Build history of the part. All positions in model axes, mm. A direction names the side the tool comes from. Round coordinates to 2 decimals unless told otherwise and drop trailing zeros. Write each loop counter-clockwise with the first axis right and the second up, starting at its lowest first coordinate (ties: lowest second). Pieces come first, ordered by that corner, then holes. Notation, with made-up numbers: (6.25, 36) -> (20.25, 36) arc R23 ccw to (20.25, 63) -> close; hole circle Ø11 at (67.5, -1.75). An arc over 180 degrees is marked (long way). Answer in a Markdown table with one row per item.
```python
from build123d import *
from build123d import SkipClean  # not in build123d's __all__

# Parameters (mm, degrees)
F1_DEPTH = 15.6
F2_R     = 4.15
F3_DEPTH = 2.1


with BuildPart() as f1:
    # F0 (on Top) → F1 (new body)
    with BuildSketch(Plane.XY):
        with BuildLine():
            ThreePointArc((-0.6628195804, -4.096726767), (0, 4.15), (0.6628195804, -4.096726767))
            Line((0.6628195804, -4.096726767), (0.6628195804, -4.25))
            Line((0.6628195804, -4.25), (15, -4.25))
            Line((15, -4.25), (15, 0))
            ThreePointArc((15, 0), (0, 15), (-15, 0))
            Line((-15, 0), (-15, -4.25))
            Line((-15, -4.25), (-0.6628195804, -4.25))
            Line((-0.6628195804, -4.25), (-0.6628195804, -4.096726767))
        make_face()
    extrude(amount=F1_DEPTH)

    # F2 (on face) → F3 (join)
    with BuildSketch(Plane(origin=(0, 0, 0), x_dir=(1, 0, 0), z_dir=(0, 0, -1))):
        with BuildLine():
            ThreePointArc((-15, 0), (0, -15), (15, 0))
            Line((15, 0), (15, 24.15))
            Line((15, 24.15), (-15, 24.15))
            Line((-15, 24.15), (-15, 0))
        make_face()
        Circle(F2_R, mode=Mode.SUBTRACT)
    with SkipClean():  # cleaning this boolean's faces spoils the solid; the shape is the same uncleaned
        extrude(amount=F3_DEPTH)


solid = f1.part
```
Q1. Saw through at C-C on z = 1.5. Write the cut outline in (x, y), plus the area to 3 significant figures.
A:
| item | result |
|---|---|
| outline | (-15, -4.25) -> (-0.66, -4.25) -> (-0.66, -4.1) arc R4.15 cw (long way) to (0.66, -4.1) -> (0.66, -4.25) -> (15, -4.25) -> (15, 0) arc R15 ccw to (-15, 0) -> close |
| area | 427 mm² |
Q2. Saw through at A-A on x = 0. Write the cut outline in (y, z), plus the area to 3 significant figures.
A:
| item | result |
|---|---|
| outline | (-24.15, -2.1) -> (-4.15, -2.1) -> (-4.15, 0) -> (-24.15, 0) -> close; (4.15, -2.1) -> (15, -2.1) -> (15, 15.6) -> (4.15, 15.6) -> close |
| area | 234 mm² |
Q3. Wall check: line 1 (Z direction, x = -9, y = -22); line 2 (Y direction, x = 0, z = 3.75); line 3 (Y direction, x = -2.5, z = 1.25). Give the ranges that are in metal, low to high. Write a range as [from, to].
A:
| item | result |
|---|---|
| line 1 | [-2.1, 0] |
| line 2 | [4.15, 15] |
| line 3 | [-4.25, -3.31], [3.31, 14.79] |
Q4. Saw through at D-D on y = -14. Write the cut outline in (x, z), plus the area to 3 significant figures.
A:
| item | result |
|---|---|
| outline | (-15, -2.1) -> (15, -2.1) -> (15, 0) -> (-15, 0) -> close |
| area | 63.0 mm² |
Q5. Which spindle directions (+Z, -Z, +X, -X, +Y, -Y) get a long thin tool onto all of the face, cutting with end or side? Do faces 1 (the flat face through (0, 6, 15.6)), 2 (the flat face through (8, -4.25, 8)). Say none if no direction does.
A:
| item | result |
|---|---|
| face 1 | +Z, +X, -X, +Y, -Y |
| face 2 | +Z, +X, -X, -Y |
Q6. Saw through at B-B on y = 3.5. Write the cut outline in (x, z).
A:
| item | result |
|---|---|
| outline | (-14.59, -2.1) -> (-2.23, -2.1) -> (-2.23, 15.6) -> (-14.59, 15.6) -> close; (2.23, -2.1) -> (14.59, -2.1) -> (14.59, 15.6) -> (2.23, 15.6) -> close |
Q7. Drop flat-ended pins along their axis: P1, Ø4.5, axis at x = 9, z = 8.5, coming from the -Y side; P2, Ø2, axis at y = -6, z = 5, coming from the -X side; P3, Ø5, axis at x = 12, z = 0, coming from the +Y side; P4, Ø6, axis at y = 4, z = 13, coming from the +X side. Give the stop position or say it passes through.
A:
| item | result |
|---|---|
| P1 | y = -4.25 |
| P2 | through |
| P3 | y = 11.61 |
| P4 | x = 14.97 |
